Build history of the part. All positions in model axes, mm. Face numbers are marked on the shaded views. Coordinates: 2 decimals unless noted, no trailing zeros. Loops run counter-clockwise (first coordinate to the right, second up) from the corner with the lowest first, then second, coordinate; pieces in that order, holes last.
(1) Wall check: L1, parallel to Y at x = -20, z = 1.6; L2, parallel to Y at x = -16, z = 0.95; L3, parallel to X at y = 17, z = 1.2. Give the ranges that are in metal, low to high.
(2) Slice it at B-B (x = 20). Give the cut face in (y, z), and give its area (3 significant figures).
(3) Slice it at C-C (z = 0.95). Give the number of separate pieces and of enclosed holes in the cut face, and give its area (3 significant figures).
(4) Two-plate mould, pull along X, no slides. Class the marked faces 1, 2 and 3: pulls with the +X half, pulls with the -X half, needs draft (parallel to the pull), parting line crosses it, or undercut.
(5) Flat gauge pin, fed straight in: P1, Ø6, axis at x = 20, y = -15, coming from the -Z side. Where does the tip first touch, or does it go through?
(6) Slice it at D-D (y = 5). Give the cut face in (x, z), and give its area (3 significant figures).
(7) Slice it at A-A (y = 23). Give the cut face in (x, z).
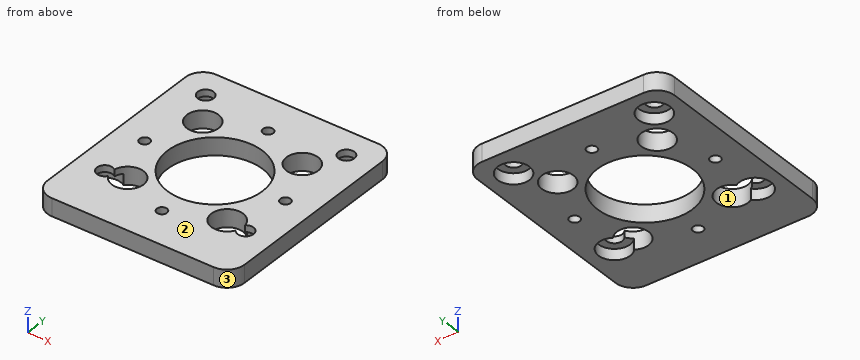
from build123d import *

# Parameters (mm, degrees)
SKETCH1_W                                        = 56
SKETCH1_H                                        = 62
SKETCH1_R                                        = 13.5
BOSS_EXTRUDE1_DEPTH                              = 5
M2_5_CLEARANCE_HOLE1_D                           = 2.9
CBORE_FOR_M4_PAN_HEAD_MACHINE_SCREW1_D           = 4.5
CBORE_FOR_M4_PAN_HEAD_MACHINE_SCREW1_CBORE_D     = 9
CBORE_FOR_M4_PAN_HEAD_MACHINE_SCREW1_CBORE_DEPTH = 3.1
FILLET1_R                                        = 5
SKETCH6_R                                        = 4.5
CUT_EXTRUDE1_DEPTH                               = 6
CUT_EXTRUDE1_DEPTH_BACK                          = 1


with BuildPart() as part:
    # Sketch1 → Boss-Extrude1 (new body)
    with BuildSketch(Plane.XY):
        Rectangle(SKETCH1_W, SKETCH1_H)
        Circle(SKETCH1_R, mode=Mode.SUBTRACT)
    extrude(amount=BOSS_EXTRUDE1_DEPTH)

    # M2.5 Clearance Hole1 (through all)
    with Locations(Plane(origin=(0, 0, 0), x_dir=(-1, 0, 0), z_dir=(0, 0, -1))):
        with Locations((0, 20), (0, -20), (20, 0), (-20, 0)):
            Hole(M2_5_CLEARANCE_HOLE1_D / 2)

    # CBORE for M4 Pan Head Machine Screw1 (through all)
    with Locations(Plane(origin=(0, 0, 0), x_dir=(-1, 0, 0), z_dir=(0, 0, -1))):
        with Locations((-20, 23), (20, 23), (20, -15), (-20, -15)):
            CounterBoreHole(CBORE_FOR_M4_PAN_HEAD_MACHINE_SCREW1_D / 2, CBORE_FOR_M4_PAN_HEAD_MACHINE_SCREW1_CBORE_D / 2, CBORE_FOR_M4_PAN_HEAD_MACHINE_SCREW1_CBORE_DEPTH)

    # Fillet1
    fillet1_edges = [part.edges().sort_by_distance(p)[0] for p in [
        (28, -31, 2.5),
        (-28, -31, 2.5),
        (-28, 31, 2.5),
        (28, 31, 2.5),
    ]]
    fillet(fillet1_edges, radius=FILLET1_R)

    # Sketch6 → Cut-Extrude1 (cut, two sides)
    with BuildSketch(Plane.XY) as cut_extrude1_sk:
        with Locations((-14.142135624, -14.142135624)):
            Circle(SKETCH6_R)
        with Locations((-14.142135624, 14.142135624)):
            Circle(SKETCH6_R)
        with Locations((14.142135624, 14.142135624)):
            Circle(SKETCH6_R)
        with Locations((14.142135624, -14.142135624)):
            Circle(SKETCH6_R)
    extrude(amount=CUT_EXTRUDE1_DEPTH, mode=Mode.SUBTRACT)
    extrude(cut_extrude1_sk.sketch, amount=-CUT_EXTRUDE1_DEPTH_BACK, mode=Mode.SUBTRACT)


solid = part.part
Response values:
1. L1: y = -31 to -19.5, -10.5 to -1.45, 1.45 to 18.5, 27.5 to 31
1. L2: y = -31 to -18.24, -10.04 to 10.04, 18.24 to 20.94, 25.06 to 31
1. L3: x = -28 to -17.62, -10.67 to 10.67, 17.62 to 28
2. outline: (-31, 0) - (-19.5, 0) - (-19.5, 3.1) - (-17.25, 3.1) - (-17.25, 5) - (-31, 5) - close; (-12.75, 3.1) - (-10.5, 3.1) - (-10.5, 0) - (-1.45, 0) - (-1.45, 5) - (-12.75, 5) - close; (1.45, 0) - (18.5, 0) - (18.5, 3.1) - (20.75, 3.1) - (20.75, 5) - (1.45, 5) - close; (25.25, 3.1) - (27.5, 3.1) - (27.5, 0) - (31, 0) - (31, 5) - (25.25, 5) - close
2. area: 223 mm2
3. separate pieces: 1
3. enclosed holes: 11
3. area: 2,370 mm2
4. face 1: undercut
4. face 2: needs draft
4. face 3: pulls with the +X half
5. P1: stops at z = 3.1
6. outline: (-28, 0) - (-12.54, 0) - (-12.54, 5) - (-28, 5) - close; (12.54, 0) - (28, 0) - (28, 5) - (12.54, 5) - close
6. area: 155 mm2
7. outline: (-28, 0) - (-24.5, 0) - (-24.5, 3.1) - (-22.25, 3.1) - (-22.25, 5) - (-28, 5) - close; (-17.75, 3.1) - (-15.5, 3.1) - (-15.5, 0) - (15.5, 0) - (15.5, 3.1) - (17.75, 3.1) - (17.75, 5) - (-17.75, 5) - close; (22.25, 3.1) - (24.5, 3.1) - (24.5, 0) - (28, 0) - (28, 5) - (22.25, 5) - close
